```python
from build123d import *

# Parameters (mm, degrees)
BOSS_EXTRUDE1_DEPTH = 17
SKETCH3_R           = 3
CUT_EXTRUDE1_DEPTH  = 45.418464629
SKETCH4_R           = 3
CUT_EXTRUDE2_DEPTH  = 45.418464629


with BuildPart() as part:
    # Sketch2 → Boss-Extrude1 (new body)
    with BuildSketch(Plane.XY):
        with BuildLine():
            Line((0, 0), (28.5, 0))
            ThreePointArc((28.5, 0), (29.560660172, 0.439339828), (30, 1.5))
            Line((30, 1.5), (30, 30))
            Line((30, 30), (28, 30))
            Line((28, 30), (28, 3.5))
            ThreePointArc((28, 3.5), (27.560660172, 2.439339828), (26.5, 2))
            Line((26.5, 2), (0, 2))
            Line((0, 2), (0, 0))
        make_face()
    extrude(amount=BOSS_EXTRUDE1_DEPTH)

    # Sketch3 → Cut-Extrude1 (cut, through all)
    with BuildSketch(Plane.ZY.offset(-28)):
        with Locations((8.5, 20)):
            Circle(SKETCH3_R)
    extrude(amount=-CUT_EXTRUDE1_DEPTH, mode=Mode.SUBTRACT)

    # Sketch4 → Cut-Extrude2 (cut, through all)
    with BuildSketch(Plane(origin=(0, 2, 0), x_dir=(1, 0, 0), z_dir=(0, 1, 0))):
        with Locations(Location((10, -8.5, 0), (0, 0, 180))):
            Circle(SKETCH4_R)
    extrude(amount=-CUT_EXTRUDE2_DEPTH, mode=Mode.SUBTRACT)


solid = part.part
```
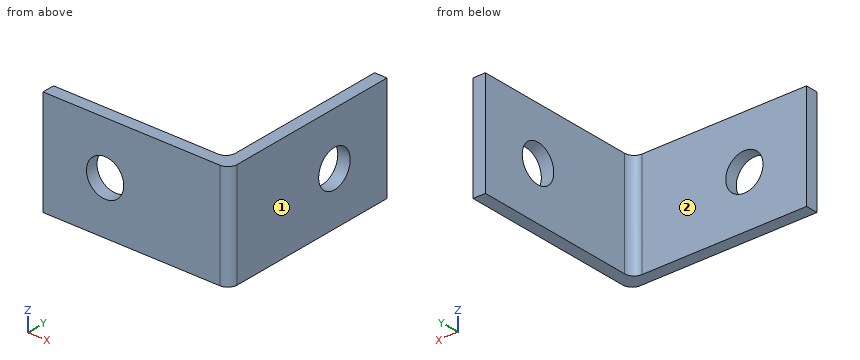
Check sheet for the modelled part. Datum: model origin and axes. Units: mm. Face numbers are marked on the shaded views. A direction names the side the tool comes from. Round coordinates to 2 decimals unless told otherwise and drop trailing zeros. Order: outer loops, then holes, each group sorted by start corner. A loop starts at its lowest first (then second) coordinate and runs counter-clockwise, first axis right, second up. Notation, with made-up numbers: (61, -3) - (115, -3) arc R31 ccw to (115, 26) - close; hole circle Ø4 at (36.5, 44.25). An arc over 180 degrees is marked (long way). Answer as CSV lines item,"result". Start each with the question number.
1) Section check A-A (z = 8.5). Record the cut outline in (x, y).
2) Scan lines: probe 1 along Y at (x, z) = (28.55, 8.5); probe 2 along Z at (x, y) = (10, 1.35); probe 3 along Y at (x, z) = (16, 3.5). Record each from-to range of solid material in increasing order.
3) Depth check by flat-ended pin: pin 1 (1.5 mm diameter, centred on x = 18.5, z = 2.5, fed in from +Y); pin 2 (1.5 mm diameter, centred on y = 26.5, z = 15, fed in from -X). Enter the tip coordinate at first touch or a pass-through.
4) Tool access check on the marked faces 1 and 2. Record the directions out of +Z, -Z, +X, -X, +Y, -Y that give a thin tool (end or side, any length) a straight path to the whole face; none if there is none.
5) Section check C-C (x = 10). Record the cut outline in (y, z).
6) Section check D-D (z = 14.25). Record the cut outline in (x, y), then the cut area to 3 significant figures.
7) Section check B-B (y = 20). Record the cut outline in (x, z).
Determined:
1,outline,"(0, 0) - (7, 0) - (7, 2) - (0, 2) - close; (13, 0) - (28.5, 0) arc R1.5 ccw to (30, 1.5) - (30, 17) - (28, 17) - (28, 3.5) arc R1.5 cw to (26.5, 2) - (13, 2) - close; (28, 23) - (30, 23) - (30, 30) - (28, 30) - close"
2,probe 1,"0 to 17, 23 to 30"
2,probe 2,"0 to 5.5, 11.5 to 17"
2,probe 3,"0 to 2"
3,pin 1,"y = 2"
3,pin 2,"x = 28"
4,face 1,"+Z, -Z, +X, +Y, -Y"
4,face 2,"+Z, -Z, -X, +Y"
5,outline,"(0, 0) - (2, 0) - (2, 5.5) - (0, 5.5) - close; (0, 11.5) - (2, 11.5) - (2, 17) - (0, 17) - close"
6,outline,"(0, 0) - (28.5, 0) arc R1.5 ccw to (30, 1.5) - (30, 30) - (28, 30) - (28, 3.5) arc R1.5 cw to (26.5, 2) - (0, 2) - close"
6,area,"116 mm^2"
7,outline,"(28, 0) - (30, 0) - (30, 5.5) - (28, 5.5) - close; (28, 11.5) - (30, 11.5) - (30, 17) - (28, 17) - close"
